For this review, use the dimensioned drawing (mm, ordinates from the lowest corner) and the shaded views. A direction names the side the tool comes from. Coordinates: 2 decimals unless noted, no trailing zeros. Write each loop counter-clockwise with the first axis right and the second up, starting at its lowest first coordinate (ties: lowest second). Pieces come first, ordered by that corner, then holes. Notation, with made-up numbers: (83, 88.25) -> (125, 88.25) arc R22 ccw to (125, 121.25) -> close; hole circle Ø10 at (-39.75, 63). An arc over 180 degrees is marked (long way). Put each result on its own line as item: value. Start each with the question number.
Item 1: For the marked faces 1, 2 and 3, list the 3-axis set-ups (+Z, -Z, +X, -X, +Y, -Y) from which the entire face can be reached by the end or side of a thin tool; tool diameter is ignored.
Item 2: To check wall thickness, follow L1, parallel to Z at x = 44, y = 6.5; L2, parallel to X at y = 27.5, z = 7.5. State the ranges of each line that lie inside material, in increasing order.
Item 3: Insertion check: P1, Ø12, axis at y = 18.5, z = 12.5, coming from the -X side; P2, Ø8, axis at y = 22, z = 13.5, coming from the +X side; P3, Ø10, axis at x = 14.5, z = 23.5, coming from the -Y side. Each pin has a flat end and moves straight along its axis. Give the tip position at first contact, or say it passes through.
Item 4: Consider section A-A on z = 8. Give the boundary of the cut face in (x, y).
Item 5: Consider section B-B on x = 51.5. Give the boundary of the cut face in (y, z), and give its area (3 significant figures).
Item 6: Consider section C-C on z = 17.5. Give the boundary of the cut face in (x, y), and give its area (3 significant figures).
Item 7: The part is to be moulded in two halves that separate along Y. For the marked faces 4, 5 and 6, say which applies: +Y half, -Y half, draft (parallel to the pull), parting line (faces both ways), or undercut.
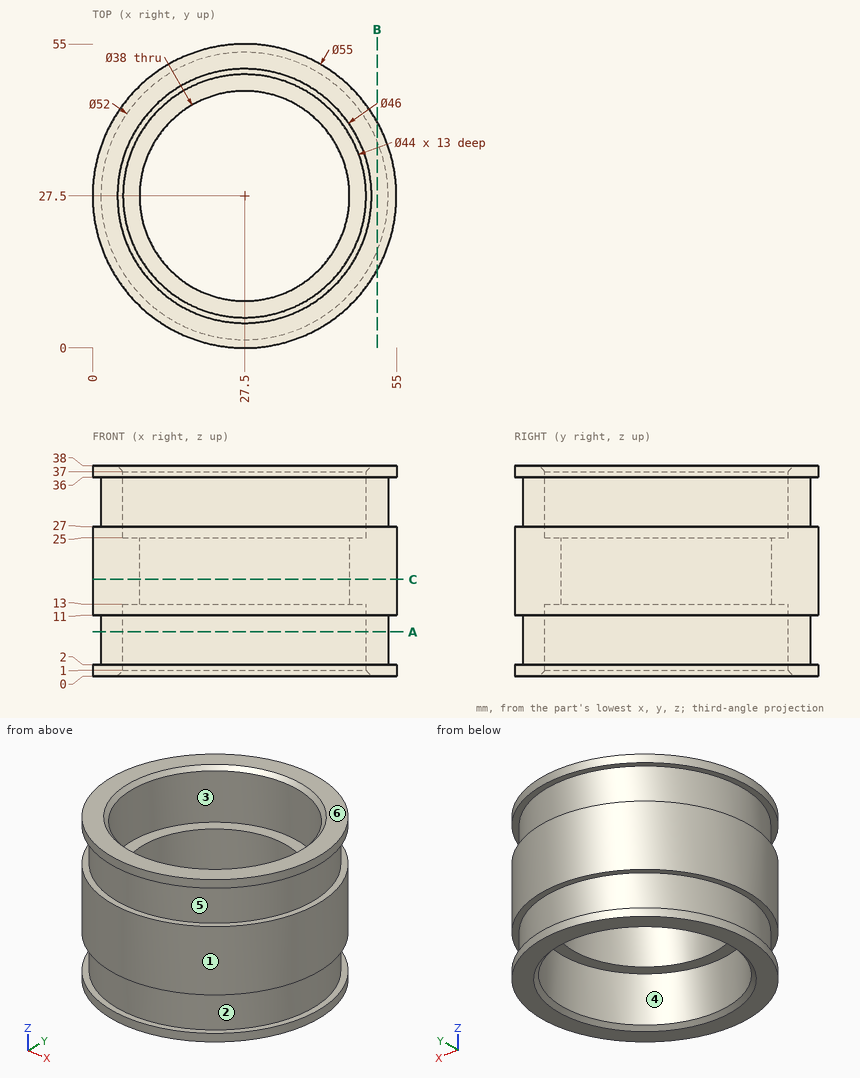
Return value:
1. face 1: +Z, -Z
1. face 2: none
1. face 3: +Z
2. L1: 0 to 2, 11 to 27, 36 to 38
2. L2: 1.5 to 5.5, 49.5 to 53.5
3. P1: x = 0.16
3. P2: x = 54.96
3. P3: y = 1.19
4. outline: circle Ø52 at (27.5, 27.5); hole circle Ø44 at (27.5, 27.5)
5. outline: (14.07, 0) -> (40.93, 0) -> (40.93, 2) -> (37.5, 2) -> (37.5, 11) -> (40.93, 11) -> (40.93, 27) -> (37.5, 27) -> (37.5, 36) -> (40.93, 36) -> (40.93, 38) -> (14.07, 38) -> (14.07, 36) -> (17.5, 36) -> (17.5, 27) -> (14.07, 27) -> (14.07, 11) -> (17.5, 11) -> (17.5, 2) -> (14.07, 2) -> close
5. area: 897 mm^2
6. outline: circle Ø55 at (27.5, 27.5); hole circle Ø38 at (27.5, 27.5)
6. area: 1,240 mm^2
7. face 4: undercut
7. face 5: parting line
7. face 6: draft
